Design review of the part built by this model. Coordinates are the model's own, in mm. A direction names the side the tool comes from. Round coordinates to 2 decimals unless told otherwise and drop trailing zeros. Write each loop counter-clockwise with the first axis right and the second up, starting at its lowest first coordinate (ties: lowest second). Pieces come first, ordered by that corner, then holes. Notation, with made-up numbers: (-15, -37.5) -> (17, -37.5) arc R11 ccw to (17, -33.5) -> close; hole circle Ø10 at (-36, 72.5). An arc over 180 degrees is marked (long way). Write item = value, one per line. Start each with the question number.
Item 1: To check wall thickness, follow L1, parallel to Z at x = 37, y = 0.8; L2, parallel to Z at x = 13, y = 2.45; L3, parallel to X at y = 1.75, z = -4. State the ranges of each line that lie inside material, in increasing order.
Item 2: Add section B-B, the plane z = -4. State the section outline as (x, y) points.
Item 3: Machinability: for faces 1 (the cylindrical face through (50.751, 3.521, -10.974)), 2 (the flat face through (30, 2, 0)), 3 (the cylindrical face through (53.66, 2.54, -25.44)), which of the approach directions +Z, -Z, +X, -X, +Y, -Y give a long, thin tool a straight path to every point of the face, cutting with its end or side? Answer none if there is none.
Item 4: Add section C-C, the plane x = 17.5. State the section outline as (y, z) points.
Item 5: Add section A-A, the plane y = 2.85. State how many separate pieces and enclosed holes the cut face has, then the cut area to 3 significant figures.
Item 6: Add section D-D, the plane z = -28.5. State the section outline as (x, y) points.
Item 7: For pin 1 Ø2.5 at (x, z) = (11, -39) entering from +Y, flat-tipped, find the tip position at first contact; note if it passes through.
Item 8: Mouldability with a two-part tool opening along Z and no side actions: class faces 4 (the flat face through (30, 3, -31.321)), 5 (the flat face through (0, 2, -30)), 6 (the cylindrical face through (2.85, 2.54, -3.01)) as released by +Z, released by -Z, zero draft, split by the parting line, or undercut.
from build123d import *

# Parameters (mm, degrees)
ESQUISSE1_W             = 60
ESQUISSE1_H             = 60
BOSS_EXTRU_1_DEPTH      = 5
ESQUISSE2_R             = 2
ESQUISSE2_R_2           = 1.3
ENL_V_MAT_EXTRU_1_DEPTH = 86
ESQUISSE4_R             = 2.5
ENL_V_MAT_EXTRU_2_DEPTH = 3
CONG_1_R                = 10
ENL_V_MAT_EXTRU_4_DEPTH = 86


with BuildPart() as part:
    # Esquisse1 → Boss.-Extru.1 (new body)
    with BuildSketch(Plane(origin=(0, 0, 0), x_dir=(1, 0, 0), z_dir=(0, 1, 0))):
        with Locations((30, 30)):
            Rectangle(ESQUISSE1_W, ESQUISSE1_H)
    extrude(amount=BOSS_EXTRU_1_DEPTH)

    # Esquisse2 → Enlèv. mat.-Extru.1 (cut, through all)
    with BuildSketch(Plane(origin=(0, 5, 0), x_dir=(1, 0, 0), z_dir=(0, 1, 0))):
        with Locations(Location((17.5, 56, 0), (0, 0, 270))):
            Circle(ESQUISSE2_R)
        with Locations(Location((17.5, 4, 0), (0, 0, 270))):
            Circle(ESQUISSE2_R)
        with Locations(Location((42.5, 4, 0), (0, 0, 270))):
            Circle(ESQUISSE2_R)
        with Locations(Location((42.5, 56, 0), (0, 0, 270))):
            Circle(ESQUISSE2_R)
        with Locations(Location((10, 38.358507613, 0), (0, 0, 270))):
            Circle(ESQUISSE2_R_2)
        with Locations(Location((10, 13.358507613, 0), (0, 0, 270))):
            Circle(ESQUISSE2_R_2)
        with Locations(Location((50, 13.358507613, 0), (0, 0, 270))):
            Circle(ESQUISSE2_R_2)
        with Locations(Location((50, 38.358507613, 0), (0, 0, 270))):
            Circle(ESQUISSE2_R_2)
    extrude(amount=-ENL_V_MAT_EXTRU_1_DEPTH, mode=Mode.SUBTRACT)

    # Esquisse4 → Enlèv. mat.-Extru.2 (cut)
    with BuildSketch(Plane(origin=(0, 5, 0), x_dir=(1, 0, 0), z_dir=(0, 1, 0))):
        with Locations(Location((10, 38.358507613, 0), (0, 0, 270))):
            Circle(ESQUISSE4_R)
        with Locations(Location((10, 13.358507613, 0), (0, 0, 270))):
            Circle(ESQUISSE4_R)
        with Locations(Location((50, 13.358507613, 0), (0, 0, 270))):
            Circle(ESQUISSE4_R)
        with Locations(Location((50, 38.358507613, 0), (0, 0, 270))):
            Circle(ESQUISSE4_R)
    extrude(amount=-ENL_V_MAT_EXTRU_2_DEPTH, mode=Mode.SUBTRACT)

    # Congé1
    cong_1_edges = [part.edges().sort_by_distance(p)[0] for p in [
        (0, 2.5, -60),
        (60, 2.5, -60),
        (60, 2.5, 0),
        (0, 2.5, 0),
    ]]
    fillet(cong_1_edges, radius=CONG_1_R)

    # Esquisse6 → Enlèv. mat.-Extru.4 (cut, through all)
    with BuildSketch(Plane(origin=(0, 5, 0), x_dir=(1, 0, 0), z_dir=(0, 1, 0))):
        with BuildLine():
            Line((15.893584332, 51.834033813), (44.106415668, 51.834033813))
            ThreePointArc((44.106415668, 51.834033813), (48.658685267, 47.281764215), (44.106415668, 42.729494617))
            Line((44.106415668, 42.729494617), (15.893584332, 42.729494617))
            ThreePointArc((15.893584332, 42.729494617), (11.341314733, 47.281764215), (15.893584332, 51.834033813))
        make_face()
        with BuildLine():
            Line((12.3529302, 31.320720192), (47.6470698, 31.320720192))
            ThreePointArc((47.6470698, 31.320720192), (53.660561739, 25.307228254), (47.6470698, 19.293736315))
            Line((47.6470698, 19.293736315), (12.3529302, 19.293736315))
            ThreePointArc((12.3529302, 19.293736315), (6.339438261, 25.307228254), (12.3529302, 31.320720192))
        make_face()
    extrude(amount=-ENL_V_MAT_EXTRU_4_DEPTH, mode=Mode.SUBTRACT)


solid = part.part
Result set:
q1.L1 = -60 to -51.83, -42.73 to -31.32, -19.29 to 0
q1.L2 = -60 to -50.8, -43.77 to -31.32, -19.29 to 0
q1.L3 = 2 to 15.5, 19.5 to 40.5, 44.5 to 58
q2.outline = (2, 0) -> (15.5, 0) -> (15.5, 5) -> (2, 5) -> close; (19.5, 0) -> (40.5, 0) -> (40.5, 5) -> (19.5, 5) -> close; (44.5, 0) -> (58, 0) -> (58, 5) -> (44.5, 5) -> close
q3.face_1 = +Y
q3.face_2 = +Z, +X, -X, +Y, -Y
q3.face_3 = +Y, -Y
q4.outline = (0, -60) -> (5, -60) -> (5, -58) -> (0, -58) -> close; (0, -54) -> (5, -54) -> (5, -51.83) -> (0, -51.83) -> close; (0, -42.73) -> (5, -42.73) -> (5, -31.32) -> (0, -31.32) -> close; (0, -19.29) -> (5, -19.29) -> (5, -6) -> (0, -6) -> close; (0, -2) -> (5, -2) -> (5, 0) -> (0, 0) -> close
q5.separate_pieces = 1
q5.enclosed_holes = 10
q5.area = 2,530 mm²
q6.outline = (0, 0) -> (7.26, 0) -> (7.26, 5) -> (0, 5) -> close; (52.74, 0) -> (60, 0) -> (60, 5) -> (52.74, 5) -> close
q7.pin_1 = 2
q8.face_4 = undercut
q8.face_5 = zero draft
q8.face_6 = released by +Z
